Autodesk Inventor part; units mm, degrees
ref_plane "YZ Plane" through (0, 0, 0) normal (1, 0, 0) x (0, 1, 0)
ref_plane "XZ Plane" through (0, 0, 0) normal (0, 1, 0) x (-1, 0, 0)
ref_plane "XY Plane" through (0, 0, 0) normal (0, 0, 1) x (1, 0, 0)
sketch "Sketch1" plane through (0, 0, 0) normal (0, 0, 1) x (1, 0, 0)
  line L0 (-47.25, -8.25) -> (47.25, -8.25)
  line L1 (47.25, -8.25) -> (47.25, 8.25)
  line L2 (47.25, 8.25) -> (-47.25, 8.25)
  line L3 (-47.25, 8.25) -> (-47.25, -8.25)
  line L4 (-47.25, -8.25) -> (47.25, 8.25) construction
  line L5 (47.25, -8.25) -> (-47.25, 8.25) construction
  point P0 (0, 0)
  dimension "d0" = 94.5
  dimension "d1" = 16.5
extrude "Extrusion1" add sketch "Sketch1" along normal blind 6
sketch "Sketch2" plane through (0, 0, 6) normal (0, 0, 1) x (1, 0, 0)
  line L0 (-19.5, 0) -> (-6.5, 0) construction
  line L1 (6.5, 0) -> (-6.5, 0) construction
  line L2 (6.5, 0) -> (19.5, 0) construction
  point P0 (0, 0)
  point P1 (0, 0)
  dimension "d4" = 13
  dimension "d5" = 13
  dimension "d6" = 13
hole "Hole1" at (-19.5, 0, 6) at (-6.5, 0, 6) at (6.5, 0, 6) at (19.5, 0, 6) direction (0, 0, -1) diameter 3.4 depth 8 tip angle 118
sketch "Sketch3" plane through (47.25, -8.25, 0) normal (1, 0, 0) x (0, 0, -1)
  line L0 (0, 0) -> (0, 16.5)
  point P0 (0, 8.25)
  point P1 (-3, 8.25)
  point P2 (0, 8.25)
  dimension "d14" = 3
hole "Hole2" at (47.25, 0, 3) direction (-1, 0, 0) diameter 2.459 depth 8.8 tip angle 118
sketch "Sketch4" plane through (-47.25, -8.25, 0) normal (-1, 0, 0) x (0, 0, 1)
  line L0 (0, 16.5) -> (0, 0)
  point P0 (0, 8.25)
  point P1 (3, 8.25)
  point P2 (0, 8.25)
  dimension "d22" = 3
hole "Hole3" at (-47.25, 0, 3) direction (1, 0, 0) diameter 2.459 depth 8.8 tip angle 118
properties part number "Kühkörper_GateTreiber" material "Aluminum 6061"
Design review of the part built by this model. Coordinates are the model's own, in mm. A direction names the side the tool comes from. Coordinates: 2 decimals unless noted, no trailing zeros. Order: outer loops, then holes, each group sorted by start corner. A loop starts at its lowest first (then second) coordinate and runs counter-clockwise, first axis right, second up. Notation, with made-up numbers: (-30, 24.5) - (27, 24.5) arc R28 ccw to (27, 51.5) - close; hole circle Ø8 at (57.25, -38). An arc over 180 degrees is marked (long way). Put each result on its own line as item: value.
1) Wall thickness on L1, parallel to X at y = 0, z = 2.8; L2, parallel to X at y = -1.5, z = 0.35: over which ranges is each line inside the solid? List them lowest first. Write a range as from..to.
Response values:
L1: x = -37.83..-21.2, -17.8..-8.2, -4.8..4.8, 8.2..17.8, 21.2..37.83
L2: x = -47.25..-20.3, -18.7..-7.3, -5.7..5.7, 7.3..18.7, 20.3..47.25
2) Take a section at B-B, the plane x = -6.5. Give the boundary of the cut face in (y, z).
Response values:
outline: (-8.25, 0) - (-1.7, 0) - (-1.7, 6) - (-8.25, 6) - close; (1.7, 0) - (8.25, 0) - (8.25, 6) - (1.7, 6) - close
3) Insertion check: P1, Ø2, axis at x = -19.5, y = 0, coming from the +Z side; P2, Ø2, axis at y = 0, z = 3, coming from the -X side. Each pin has a flat end and moves straight along its axis. Give the tip position at first contact, or say it passes through.
Response values:
P1: passes through
P2: stops at x = -38.31
4) Take a section at A-A, the plane x = -40. Give the boundary of the cut face in (y, z).
Response values:
outline: (-8.25, 0) - (8.25, 0) - (8.25, 6) - (-8.25, 6) - close; hole circle Ø2.46 at (0, 3)
5) The part is to be moulded in two halves that separate along X. For faces 1 (the face through (37.84, 0.009, 3.213)), 2 (the face through (-21.186, 0.221, 2.958)), 3 (the face through (42.788, -0.369, 1.827)), say which applies: released by +X, released by -X, zero draft, split by the parting line, or undercut.
Response values:
face 1: released by +X
face 2: undercut
face 3: zero draft
6) Tool access review of faces 4 (the face through (-42.79, 1.09, 3.57)), 5 (the face through (-47.25, 0.1, 1.6)): name each direction out of +Z, -Z, +X, -X, +Y, -Y from which nothing blocks a thin tool from reaching the whole face with its end or side.
Response values:
face 4: -X
face 5: +Z, -Z, -X, +Y, -Y
